Drawing for the job (mm, zero at the part's lowest x, y, z). Round coordinates to 2 decimals unless told otherwise and drop trailing zeros. Loops run counter-clockwise (first coordinate to the right, second up) from the corner with the lowest first, then second, coordinate; pieces in that order, holes last. Notation, with made-up numbers: (69.25, 25) -> (124.25, 25) arc R5 cw to (124.25, 32) -> close; hole circle Ø10 at (85.5, 29.25). An arc over 180 degrees is marked (long way). Put each result on its own line as item: value. Start each with the question number.
Item 1: Pull direction Y, two halves, no side cores. Call the marked faces 1, 2 and 3: +Y half, -Y half, draft (parallel to the pull), parting line (faces both ways), or undercut.
Item 2: Drill centre lines: probe 1 along Z at (x, y) = (28, 5); probe 2 along Z at (x, y) = (4, 3); probe 3 along X at (y, z) = (21.5, 29). Where is each one in solid material? Low to high. Write a range as [from, to].
Item 3: Cut at D-D, the plane x = 27. List the corners of the cut face in (y, z).
Item 4: Flat gauge pin, fed straight in: pin 1 Ø3.5 at (x, z) = (28, 40.5) entering from -Y. Where does the tip first touch, or does it go through?
Item 5: Cut at A-A, the plane x = 16. List the corners of the cut face in (y, z), plus the area to 3 significant figures.
Item 6: Cut at C-C, the plane z = 40.5. List the corners of the cut face in (x, y).
Item 7: Cut at B-B, the plane y = 27. List the corners of the cut face in (x, z).
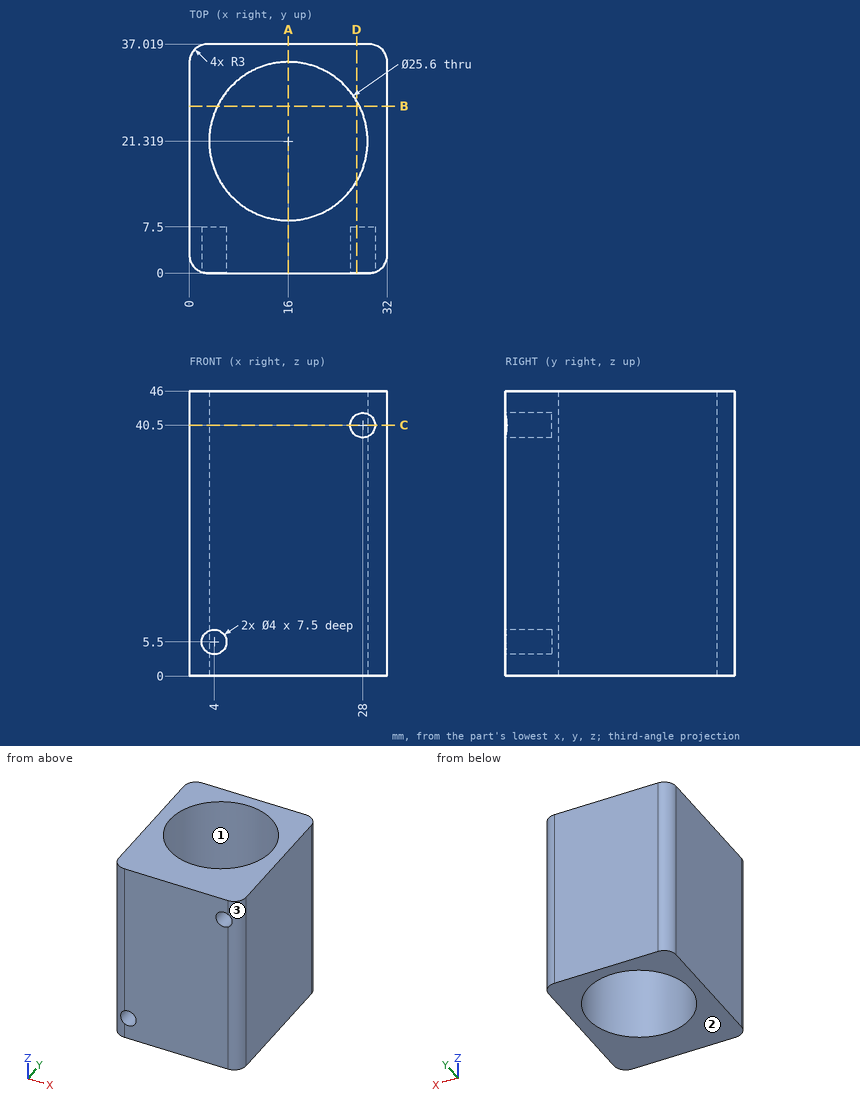
Reply:
1. face 1: undercut
1. face 2: draft
1. face 3: -Y half
2. probe 1: z = [0, 38.5], [42.5, 46]
2. probe 2: z = [0, 3.5], [7.5, 46]
2. probe 3: x = [0, 3.2], [28.8, 32]
3. outline: (0, 0) -> (14.77, 0) -> (14.77, 46) -> (0, 46) -> (0, 42.23) -> (7.5, 42.23) -> (7.5, 38.77) -> (0, 38.77) -> close; (27.86, 0) -> (37.02, 0) -> (37.02, 46) -> (27.86, 46) -> close
4. pin 1: stops at y = 7.5
5. outline: (0, 0) -> (8.52, 0) -> (8.52, 46) -> (0, 46) -> close; (34.12, 0) -> (37.02, 0) -> (37.02, 46) -> (34.12, 46) -> close
5. area: 525 mm^2
6. outline: (0, 3) arc R3 ccw to (3, 0) -> (26, 0) -> (26, 7.5) -> (30, 7.5) -> (30, 0.17) arc R3 ccw to (32, 3) -> (32, 34.02) arc R3 ccw to (29, 37.02) -> (3, 37.02) arc R3 ccw to (0, 34.02) -> close; hole circle Ø25.6 at (16, 21.32)
7. outline: (0, 0) -> (4.53, 0) -> (4.53, 46) -> (0, 46) -> close; (27.47, 0) -> (32, 0) -> (32, 46) -> (27.47, 46) -> close
